from build123d import *

# Parameters (mm, degrees)
BOSS_EXTRUDE1_DEPTH     = 60
FILLET1_R               = 6
SKETCH2_R               = 2.05
CUT_EXTRUDE1_DEPTH      = 62.318838867
LPATTERN1_COUNT         = 4
LPATTERN1_PITCH         = 8
MIRROR1_COPY_1_SKETCH_R = 2.05
MIRROR1_COPY_1_DEPTH    = 62.318838867
MIRROR1_COPY_2_SKETCH_R = 2.05
MIRROR1_COPY_2_DEPTH    = 62.318838867
MIRROR1_COPY_3_SKETCH_R = 2.05
MIRROR1_COPY_3_DEPTH    = 62.318838867


with BuildPart() as part:
    # Sketch1 → Boss-Extrude1 (new body)
    with BuildSketch(Plane.XY):
        Polygon((0, 0), (4, 0), (4, 2), (3, 2), (3, 10), (4, 10), (4, 12), (0, 12), align=None)
    extrude(amount=-BOSS_EXTRUDE1_DEPTH)

    # Fillet1
    fillet1_edges = [part.edges().sort_by_distance(p)[0] for p in [
        (2, 12, 0),
        (2, 0, 0),
        (2, 0, -60),
        (2, 12, -60),
    ]]
    fillet(fillet1_edges, radius=FILLET1_R - 0.0001)  # a hair under: the kernel refuses the full size

    # Sketch2 → Cut-Extrude1 (cut, through all)
    with BuildSketch(Plane.ZY):
        with Locations(Location((-54, 6, 0), (0, 0, 270))):
            Circle(SKETCH2_R)
    cut_extrude1 = extrude(amount=-CUT_EXTRUDE1_DEPTH, mode=Mode.SUBTRACT)

    # LPattern1: Cut-Extrude1 ×4
    with Locations(*[(0, 0, i * LPATTERN1_PITCH) for i in range(1, LPATTERN1_COUNT)]):
        add(cut_extrude1, mode=Mode.SUBTRACT)

    # Mirror1: Cut-Extrude1 across plane
    add(cut_extrude1.mirror(Plane.XY.offset(-30)), mode=Mode.SUBTRACT)

    # Mirror1 copy 1 sketch → Mirror1 copy 1 (cut, through all)
    with BuildSketch(Plane(origin=(0, 0, -68), x_dir=(0, 0, -1), z_dir=(-1, 0, 0))):
        with Locations((-54, -6)):
            Circle(MIRROR1_COPY_1_SKETCH_R)
    extrude(amount=-MIRROR1_COPY_1_DEPTH, mode=Mode.SUBTRACT)

    # Mirror1 copy 2 sketch → Mirror1 copy 2 (cut, through all)
    with BuildSketch(Plane(origin=(0, 0, -76), x_dir=(0, 0, -1), z_dir=(-1, 0, 0))):
        with Locations((-54, -6)):
            Circle(MIRROR1_COPY_2_SKETCH_R)
    extrude(amount=-MIRROR1_COPY_2_DEPTH, mode=Mode.SUBTRACT)

    # Mirror1 copy 3 sketch → Mirror1 copy 3 (cut, through all)
    with BuildSketch(Plane(origin=(0, 0, -84), x_dir=(0, 0, -1), z_dir=(-1, 0, 0))):
        with Locations((-54, -6)):
            Circle(MIRROR1_COPY_3_SKETCH_R)
    extrude(amount=-MIRROR1_COPY_3_DEPTH, mode=Mode.SUBTRACT)


solid = part.part
Build history of the part. All positions in model axes, mm. A direction names the side the tool comes from. Give positions to 0.01 mm unless a question says otherwise; leave off trailing zeros. Order: outer loops, then holes, each group sorted by start corner. A loop starts at its lowest first (then second) coordinate and runs counter-clockwise, first axis right, second up. Notation, with made-up numbers: M 88.25,9.25 L 123.25,9.25 A20 cw 123.25,32.25 Z; hole C 55,21 d6. An arc over 180 degrees is marked long. Use one line per item in the form item = value.
Q1. Which spindle directions (+Z, -Z, +X, -X, +Y, -Y) get a long thin tool onto all of the face, cutting with end or side? Do faces 5 (the flat face through (3.5, 10, -29.6)), 6 (the cylindrical face through (1.479, 6.267, -51.967)). Say none if no direction does.
Conclusion:
face_5 = +Z, -Z, +X
face_6 = +X, -X
Q2. Pin check, flat tips, straight feed: P1, Ø1.5, axis at x = 2, y = 7, coming from the -Z side; P2, Ø3.5, axis at y = 6, z = -22, coming from the +X side (3 decimals); P3, Ø4.5, axis at y = 6, z = -30, coming from the +X side. Stop position of each tip, or through.
Conclusion:
P1 = -59.99
P2 = through
P3 = 3
Q3. Slice it at C-C, the plane z = -31. Write the cut outline in (x, y).
Conclusion:
outline = M 0,0 L 4,0 L 4,2 L 3,2 L 3,4.21 L 0,4.21 Z; M 0,7.79 L 3,7.79 L 3,10 L 4,10 L 4,12 L 0,12 Z
Q4. Slice it at B-B, the plane x = 1.95. State how many separate pieces and enclosed holes the cut face has, and give its area (3 significant figures).
Conclusion:
separate_pieces = 1
enclosed_holes = 7
area = 597 mm2
Q5. Wall check: probe 1 along Y at (x, z) = (3.5, -12); probe 2 along X at (y, z) = (3.25, -14); probe 3 along Y at (x, z) = (2.35, -22). Give the ranges that are in metal, low to high.
Conclusion:
probe_1 = 0 to 2, 10 to 12
probe_2 = 0 to 3
probe_3 = 0 to 3.95, 8.05 to 12
Q6. Slice it at A-A, the plane z = -46. Write the cut outline in (x, y).
Conclusion:
outline = M 0,0 L 4,0 L 4,2 L 3,2 L 3,3.95 L 0,3.95 Z; M 0,8.05 L 3,8.05 L 3,10 L 4,10 L 4,12 L 0,12 Z
Q7. Pull direction Z, two halves, no side cores. Call faces 1 (the cylindrical face through (2.028, 1.711, -58.196)), 2 (the flat face through (4, 11, -30)), 3 (the cylindrical face through (1.479, 6.267, -35.967)), 4 (the cylindrical face through (1.972, 10.289, -1.804)): released by +Z, released by -Z, zero draft, split by the parting line, or undercut.
Conclusion:
face_1 = released by -Z
face_2 = zero draft
face_3 = undercut
face_4 = released by +Z
Q8. Slice it at D-D, the plane y = 9. Write the cut outline in (x, z).
Conclusion:
outline = M 0,-59.2 L 3,-59.2 L 3,-0.8 L 0,-0.8 Z
